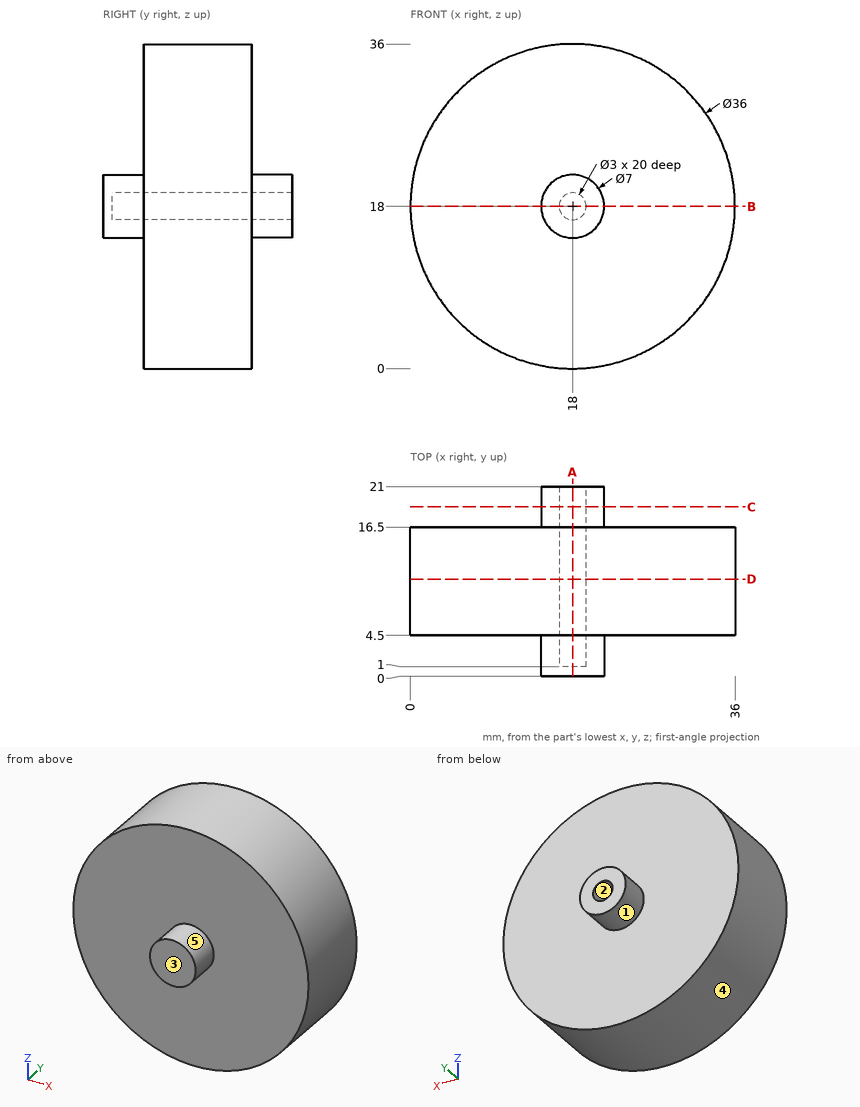
Geometry: see drawing. Coordinates: mm, zero at the bounding-box minimum. A direction names the side the tool comes from. Coordinates: 2 decimals unless noted, no trailing zeros. Write each loop counter-clockwise with the first axis right and the second up, starting at its lowest first coordinate (ties: lowest second). Pieces come first, ordered by that corner, then holes.
1) Section A-A on x = 18. Output: boundary loops of the cut face in (y, z).
2) Set-up query: the marked faces 4 and 5. Return all of +Z, -Z, +X, -X, +Y, -Y with unobstructed straight access to the full face (end or side cutting, diameter ignored); none if empty.
3) Section B-B on z = 18. Output: boundary loops of the cut face in (x, y), and give its area (3 significant figures).
4) Section D-D on y = 10.75. Output: boundary loops of the cut face in (x, z).
5) Pin query (flat end, axial travel): pin 1 Ø1 at (x, z) = (14, 9.5) entering from +Y; pin 2 Ø10 at (y, z) = (2, 27.5) entering from +X; pin 3 Ø10 at (x, y) = (8.5, 14) entering from -Z. Return the tip coordinate at first contact, or that it passes through.
6) Material intervals for line 1 along Z through (x, y) = (18, 11); line 2 along Z through (x, y) = (18, 16.75); line 3 along Y through (x, z) = (18.5, 4), sorted ascending.
7) Mould query, pull axis X, two halves, no side actions, for the marked faces 1, 2 and 3. Classes: pulls with the +X half, pulls with the -X half, needs draft (parallel to the pull), parting line crosses it, or undercut.
8) Section C-C on y = 18.75. Output: boundary loops of the cut face in (x, z).
Check result:
1. outline: (0, 14.5) - (4.5, 14.5) - (4.5, 0) - (16.5, 0) - (16.5, 14.5) - (21, 14.5) - (21, 16.5) - (1, 16.5) - (1, 19.5) - (21, 19.5) - (21, 21.5) - (16.5, 21.5) - (16.5, 36) - (4.5, 36) - (4.5, 21.5) - (0, 21.5) - close
2. face 4: +Y, -Y
2. face 5: -Y
3. outline: (0, 4.5) - (14.5, 4.5) - (14.5, 0) - (21.5, 0) - (21.5, 4.5) - (36, 4.5) - (36, 16.5) - (21.5, 16.5) - (21.5, 21) - (19.5, 21) - (19.5, 1) - (16.5, 1) - (16.5, 21) - (14.5, 21) - (14.5, 16.5) - (0, 16.5) - close
3. area: 435 mm2
4. outline: circle Ø36 at (18, 18); hole circle Ø3 at (18, 18)
5. pin 1: stops at y = 16.5
5. pin 2: stops at x = 35.24
5. pin 3: stops at z = 0.57
6. line 1: z = 0 to 16.5, 19.5 to 36
6. line 2: z = 14.5 to 16.5, 19.5 to 21.5
6. line 3: y = 4.5 to 16.5
7. face 1: parting line crosses it
7. face 2: undercut
7. face 3: needs draft
8. outline: circle Ø7 at (18, 18); hole circle Ø3 at (18, 18)
